```python
from build123d import *

# Parameters (mm, degrees)
F1_DEPTH = 50.8
F3_D     = 6.35


with BuildPart() as f1:
    # F0 (on Right) → F1 (new body)
    with BuildSketch(Plane.YZ):
        with BuildLine():
            Line((0, 133.35), (0, 0))
            ThreePointArc((0, 0), (20.205576, 8.369424), (28.575, 28.575))
            Line((28.575, 28.575), (28.575, 133.35))
            Line((28.575, 133.35), (0, 133.35))
        make_face()
    extrude(amount=F1_DEPTH)

    # F3 (through all)
    with Locations(Plane.YZ.offset(50.8)):
        with Locations((19.05, 120.65)):
            Hole(F3_D / 2)


solid = f1.part
```
Work out the finished part from the listing and answer in its coordinate system (mm). Give positions to 0.01 mm unless a question says otherwise; leave off trailing zeros. Loops run counter-clockwise (first coordinate to the right, second up) from the corner with the lowest first, then second, coordinate; pieces in that order, holes last. Notation, with made-up numbers: (20.25, -2.5) - (53.25, -2.5) arc R14 cw to (53.25, 12.5) - close; hole circle Ø6 at (71, 66). An arc over 180 degrees is marked (long way). One line per question, with ' | ' between items.
(1) Each of these flat-tipped pins is pushed along its axis until it touches: pin 1 Ø3 at (x, y) = (36, 24.5) entering from -Z; pin 2 Ø8 at (x, y) = (17.5, 12.5) entering from -Z; pin 3 Ø8 at (x, y) = (45, 15) entering from -Z. Where does it stop, or does it pass through?
Recorded:
pin 1: stops at z = 11.62 | pin 2: stops at z = 1.29 | pin 3: stops at z = 2.2
(2) The part is cut by section B-B (x = 34.5). Write down the section's boundary in (y, z) (3 decimals).
Recorded:
outline: (0, 0) arc R28.575 ccw to (28.575, 28.575) - (28.575, 133.35) - (0, 133.35) - close; hole circle Ø6.35 at (19.05, 120.65)
(3) Straight lines are drawn through the part: probe 1 along Z at (x, y) = (35.5, 19.05) (3 decimals); probe 2 along Y at (x, z) = (35, 120) (3 decimals); probe 3 along Z at (x, y) = (5.5, 1.5). For each, find the intervals that lie inside material, in ascending order.
Recorded:
probe 1: z = 7.276 to 117.475, 123.825 to 133.35 | probe 2: y = 0 to 15.942, 22.158 to 28.575 | probe 3: z = 0.04 to 133.35
(4) The part is cut by section D-D (y = 26). Write down the section's boundary in (x, z).
Recorded:
outline: (0, 16.72) - (50.8, 16.72) - (50.8, 133.35) - (0, 133.35) - close
(5) The part is cut by section C-C (y = 20). Write down the section's boundary in (x, z).
Recorded:
outline: (0, 8.17) - (50.8, 8.17) - (50.8, 117.62) - (0, 117.62) - close; (0, 123.68) - (50.8, 123.68) - (50.8, 133.35) - (0, 133.35) - close
(6) The part is cut by section A-A (z = 120.65). Write down the section's boundary in (x, y) (3 decimals), then the cut area to 3 significant figures.
Recorded:
outline: (0, 0) - (50.8, 0) - (50.8, 15.875) - (0, 15.875) - close; (0, 22.225) - (50.8, 22.225) - (50.8, 28.575) - (0, 28.575) - close | area: 1,130 mm²
(7) The mould has two halves that part along Y. Classify faces 1 (the face through (25, 14, 133.35)), 2 (the face through (25.04, 19.74, 117.55)), 3 (the face through (25, 0, 68)), 4 (the face through (25, 28.575, 80)): +Y half, -Y half, draft (parallel to the pull), parting line (faces both ways), or undercut.
Recorded:
face 1: draft | face 2: undercut | face 3: -Y half | face 4: +Y half
